```python
from build123d import *

# Parameters (mm, degrees)
F0_R     = 4.75
F1_DEPTH = 45
F2_R     = 1.75
F3_DEPTH = 1
F4_R     = 0.8
F5_R     = 1


with BuildPart() as f1:
    # F0 (on Top) → F1 (new body)
    with BuildSketch(Plane.XY):
        Circle(F0_R)
    extrude(amount=F1_DEPTH)

    # F2 (on face) → F3 (join)
    with BuildSketch(Plane.XY.offset(45)):
        Circle(F2_R)
    extrude(amount=F3_DEPTH)

    # F4
    f4_edges = [f1.edges().sort_by_distance(p)[0] for p in [
        (-1.75, 0, 46),
    ]]
    fillet(f4_edges, radius=F4_R)

    # F5
    f5_edges = [f1.edges().sort_by_distance(p)[0] for p in [
        (-4.75, 0, 45),
        (-4.75, 0, 0),
    ]]
    fillet(f5_edges, radius=F5_R)


solid = f1.part
```
Work out the finished part from the listing and answer in its coordinate system (mm). A direction names the side the tool comes from. Give positions to 0.01 mm unless a question says otherwise; leave off trailing zeros. Loops run counter-clockwise (first coordinate to the right, second up) from the corner with the lowest first, then second, coordinate; pieces in that order, holes last. Notation, with made-up numbers: (45.25, -39) -> (74.25, -39) arc R16 cw to (74.25, -21) -> close; hole circle Ø2 at (84.5, 3.25). An arc over 180 degrees is marked (long way). Use CSV: the item, a comma, the result in double quotes.
1. The part is cut by section C-C (z = 28.5). Write down the section's boundary in (x, y), then the cut area to 3 significant figures.
Found:
outline,"circle Ø9.5 at (0, 0)"
area,"70.9 mm^2"
2. The part is cut by section A-A (y = 0). Write down the section's boundary in (x, z), then the cut area to 3 significant figures.
Found:
outline,"(-4.75, 1) arc R1 ccw to (-3.75, 0) -> (3.75, 0) arc R1 ccw to (4.75, 1) -> (4.75, 44) arc R1 ccw to (3.75, 45) -> (1.75, 45) -> (1.75, 45.2) arc R0.8 ccw to (0.95, 46) -> (-0.95, 46) arc R0.8 ccw to (-1.75, 45.2) -> (-1.75, 45) -> (-3.75, 45) arc R1 ccw to (-4.75, 44) -> close"
area,"430 mm^2"
3. Straight lines are drawn through the part: line 1 (Z direction, x = -0.25, y = 2); line 2 (Y direction, x = -0.25, z = 42); line 3 (Y direction, x = -1.25, z = 31.5). For each, find the intervals that lie inside material, in ascending order.
Found:
line 1,"0 to 45"
line 2,"-4.74 to 4.74"
line 3,"-4.58 to 4.58"
4. A tool of negligible diameter and unlimited length cuts with its end or side. For faces 3 (the flat face through (0, 0, 0)), 4 (the flat face through (2, -1, 45)), from which of +Z, -Z, +X, -X, +Y, -Y can it reach the whole face along a straight path? Write none if from no direction.
Found:
face 3,"-Z, +X, -X, +Y, -Y"
face 4,"+Z"
5. Flat-ended cylindrical pins translate along their axes: pin 1 Ø1 at (y, z) = (3.5, 34) entering from -X; pin 2 Ø1 at (x, y) = (-1, 3) entering from +Z; pin 3 Ø5 at (y, z) = (-3.5, 5.5) entering from +X. Find the tip coordinate at first contact, or state that the pin passes through.
Found:
pin 1,"x = -3.68"
pin 2,"z = 45"
pin 3,"x = 4.64"
6. The mould has two halves that part along X. Classify faces 1 (the cylindrical face through (2.192, -4.214, 22.199)), 2 (the flat face through (0, 0, 46)): +X half, -X half, draft (parallel to the pull), parting line (faces both ways), or undercut.
Found:
face 1,"parting line"
face 2,"draft"
